The model under review builds one solid part; all positions refer to its coordinate system, in mm. Face numbers are marked on the shaded views. A direction names the side the tool comes from. Coordinates: 2 decimals unless noted, no trailing zeros. Loops run counter-clockwise (first coordinate to the right, second up) from the corner with the lowest first, then second, coordinate; pieces in that order, holes last. Notation, with made-up numbers: (46.5, -6) -> (95.5, -6) arc R10 cw to (95.5, 12) -> close; hole circle Ø6 at (37.25, 32.25). An arc over 180 degrees is marked (long way). One line per question, with ' | ' between items. Start each with the question number.
from build123d import *

# Parameters (mm, degrees)
F0_W     = 50.8
F0_H     = 76.2
F1_DEPTH = 101.6
F3_DEPTH = 50.801
F4_T     = -1.905
F5_W     = 25.4
F5_H     = 19.05
F6_DEPTH = 3.048


with BuildPart() as f1:
    # F0 (on Front) → F1 (new body)
    with BuildSketch(Plane.XZ):
        with Locations((25.4, 38.1)):
            Rectangle(F0_W, F0_H)
    extrude(amount=F1_DEPTH)

    # F2 (on face) → F3 (cut, through all)
    with BuildSketch(Plane.YZ.offset(50.8)):
        Polygon((-101.6, 0), (0, 0), (0, 12.7), align=None)
    extrude(amount=-F3_DEPTH, mode=Mode.SUBTRACT)

    # F4
    f4_openings = [f1.faces().sort_by_distance(p)[0] for p in [
        (25.4, -50.8, 76.2),
    ]]
    offset(amount=F4_T, openings=f4_openings)

    # F5 (on face) → F6 (cut)
    with BuildSketch(Plane(origin=(0, -1.563077, 12.504615), x_dir=(1, 0, 0), z_dir=(0, 0.124035, -0.992278))):
        with Locations((25.4, 88.750432)):
            Rectangle(F5_W, F5_H)
    extrude(amount=-F6_DEPTH, mode=Mode.SUBTRACT)


solid = f1.part
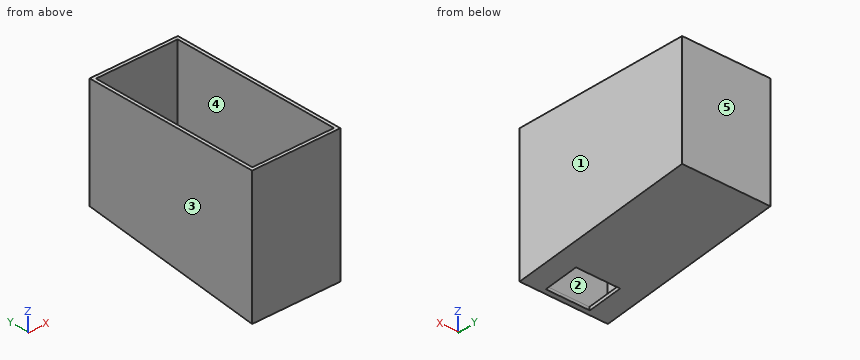
1) Machinability: for the marked faces 1 and 2, which of the approach directions +Z, -Z, +X, -X, +Y, -Y give a long, thin tool a straight path to every point of the face, cutting with its end or side? Answer none if there is none.
2) Consider section B-B, the plane z = 31. Write out the cut boundary in (x, y) (3 decimals).
3) Consider section A-A, the plane x = 28. Write out the cut boundary in (y, z) (3 decimals).
4) Consider section D-D, the plane x = 8.5. Write out the cut boundary in (y, z) (3 decimals).
5) Wall thickness on L1, parallel to X at y = -23, z = 18 (3 decimals); L2, parallel to Y at x = 38, z = 23.5 (3 decimals); L3, parallel to Z at x = 36.5, y = -42: over which ranges is each line inside the solid? List them lowest first.
6) Consider section C-C, the plane y = -92. Write out the cut boundary in (x, z) (3 decimals).
7) Insertion check: pin 1 Ø1 at (x, y) = (24.5, -54) entering from -Z; pin 2 Ø12 at (x, y) = (38, -34) entering from -Z; pin 3 Ø1.5 at (x, y) = (21.5, -73) entering from +Z. Each pin has a flat end and moves straight along its axis. Give the tip position at first contact, or say it passes through.
8) Mouldability with a two-part tool opening along X and no side actions: class the marked faces 3, 4 and 5 as +X half, -X half, draft (parallel to the pull), parting line (faces both ways), or undercut.
Filled sheet:
1) face 1: +Z, -Z, +X, +Y, -Y | face 2: +Z
2) outline: (0, -101.6) -> (50.8, -101.6) -> (50.8, 0) -> (0, 0) -> close; hole (1.905, -99.695) -> (48.895, -99.695) -> (48.895, -1.905) -> (1.905, -1.905) -> close
3) outline: (-101.6, 0) -> (-99.08, 0.315) -> (-99.316, 2.205) -> (-99.695, 2.158) -> (-99.695, 76.2) -> (-101.6, 76.2) -> close; (-80.413, 4.568) -> (-80.177, 2.678) -> (0, 12.7) -> (0, 76.2) -> (-1.905, 76.2) -> (-1.905, 14.382) -> close
4) outline: (-101.6, 0) -> (0, 12.7) -> (0, 76.2) -> (-1.905, 76.2) -> (-1.905, 14.382) -> (-99.695, 2.158) -> (-99.695, 76.2) -> (-101.6, 76.2) -> close
5) L1: 0 to 1.905, 48.895 to 50.8 | L2: -101.6 to -99.695, -1.905 to 0 | L3: 7.45 to 9.37
6) outline: (0, 1.2) -> (12.7, 1.2) -> (12.7, 3.12) -> (1.905, 3.12) -> (1.905, 76.2) -> (0, 76.2) -> close; (38.1, 1.2) -> (50.8, 1.2) -> (50.8, 76.2) -> (48.895, 76.2) -> (48.895, 3.12) -> (38.1, 3.12) -> close
7) pin 1: z = 5.89 | pin 2: z = 7.7 | pin 3: z = 5.59
8) face 3: -X half | face 4: undercut | face 5: draft
